Check sheet for the modelled part. Datum: model origin and axes. Units: mm. A direction names the side the tool comes from. Coordinates: 2 decimals unless noted, no trailing zeros. Order: outer loops, then holes, each group sorted by start corner. A loop starts at its lowest first (then second) coordinate and runs counter-clockwise, first axis right, second up. Notation, with made-up numbers: M 40,37 L 87,37 A26 cw 87,53 Z; hole C 48,-30 d10. An arc over 180 degrees is marked long. Answer in a Markdown table with one row per item. Add a question column.
from build123d import *

# Parameters (mm, degrees)
SKETCH_1_W      = 10
SKETCH_1_H      = 10
SKETCH_1_W_2    = 8
SKETCH_1_H_2    = 8
EXTRUDE_1_DEPTH = 155


with BuildPart() as part:
    # 草图1 → 凸台-拉伸1 (new body)
    with BuildSketch(Plane.XZ.offset(155)):
        with Locations((40, 0)):
            Rectangle(SKETCH_1_W, SKETCH_1_H)
        with Locations((40, 0)):
            Rectangle(SKETCH_1_W_2, SKETCH_1_H_2, mode=Mode.SUBTRACT)
    extrude(amount=-EXTRUDE_1_DEPTH)


solid = part.part
1. Section check B-B on y = -144. Enter the section's corners in (x, z), then the cut area to 3 significant figures.
2. Set-up check for faces 1 (the flat face through (40, -79, -5)), 2 (the flat face through (36, -79, 0)): record each of +Z, -Z, +X, -X, +Y, -Y from which the full face is reachable in a straight line by a thin tool's end or side.
3. Section check A-A on x = 41. Enter the section's corners in (y, z), then the cut area to 3 significant figures.
4. Section check C-C on z = 2.5. Enter the section's corners in (x, y).
5. Scan lines: line 1 (Z direction, x = 43.5, y = -94); line 2 (X direction, y = -65.5, z = -1). Record each from-to range of solid material in increasing order.
Result sheet:
| question | item | result |
|---|---|---|
| 1 | outline | M 35,-5 L 45,-5 L 45,5 L 35,5 Z; hole M 36,-4 L 44,-4 L 44,4 L 36,4 Z |
| 1 | area | 36.0 mm^2 |
| 2 | face 1 | -Z, +X, -X, +Y, -Y |
| 2 | face 2 | +Y, -Y |
| 3 | outline | M -155,-5 L 0,-5 L 0,-4 L -155,-4 Z; M -155,4 L 0,4 L 0,5 L -155,5 Z |
| 3 | area | 310 mm^2 |
| 4 | outline | M 35,-155 L 36,-155 L 36,0 L 35,0 Z; M 44,-155 L 45,-155 L 45,0 L 44,0 Z |
| 5 | line 1 | -5 to -4, 4 to 5 |
| 5 | line 2 | 35 to 36, 44 to 45 |
